```python
from build123d import *

# Parameters (mm, degrees)
F0_W     = 63.5
F0_H     = 63.5
F1_DEPTH = 3.175
F3_DEPTH = 25.4
F4_R     = 1.524
F6_D     = 8.4328


with BuildPart() as f1:
    # F0 (on Top) → F1 (new body)
    with BuildSketch(Plane.XY):
        with Locations((31.75, 31.75)):
            Rectangle(F0_W, F0_H)
    extrude(amount=F1_DEPTH)

    # F2 (on face) → F3 (join)
    with BuildSketch(Plane.XY.offset(3.175)):
        with BuildLine():
            ThreePointArc((31.75, 21.8313), (34.27345197, 22.87654803), (35.3187, 25.4))
            ThreePointArc((35.3187, 25.4), (29.22654803, 27.92345197), (31.75, 21.8313))
        make_face()
    extrude(amount=F3_DEPTH)

    # F4
    f4_edges = [f1.edges().sort_by_distance(p)[0] for p in [
        (31.75, 28.9687, 28.575),
    ]]
    fillet(f4_edges, radius=F4_R)

    # F6 (through all)
    with Locations(Plane.XY.offset(3.175)):
        with Locations((16.5602006018, 19.0660767257), (51.1259697378, 19.6664221585)):
            Hole(F6_D / 2)


solid = f1.part
```
Work out the finished part from the listing and answer in its coordinate system (mm). Round coordinates to 2 decimals unless told otherwise and drop trailing zeros. Loops run counter-clockwise (first coordinate to the right, second up) from the corner with the lowest first, then second, coordinate; pieces in that order, holes last. Notation, with made-up numbers: (68, 34.25) -> (123, 34.25) arc R21 ccw to (123, 53.25) -> close; hole circle Ø8 at (5.25, 34.25). An arc over 180 degrees is marked (long way). Write each question's results on one line, items separated by ' | '. Start each with the question number.
1. For a pull along X with two mould halves and no side action, classify faces 1 (the face through (31, 0, 2)), 2 (the face through (12.665, 17.451, 1.565)), 3 (the face through (63.5, 31, 2)) as +X half, -X half, draft (parallel to the pull), parting line (faces both ways), or undercut.
2. Section C-C (y = 32.5) is taken. Determine the outline of the cut face in (x, z) (3 decimals), plus the area to 3 significant figures.
3. Given pin 1 Ø3 at (y, z) = (9.5, 5.5) entering from -X; pin 2 Ø13.5 at (x, y) = (51.13, 19.67) entering from -Z; pin 3 Ø4 at (x, y) = (56, 19.5) entering from +Z (3 decimals); pin 4 Ø4 at (y, z) = (21.5, 9.5) entering from -X, each flat-ended and moving along its own axis, determine where each tip first touches the part or whether it passes through.
4. Find the intervals of material crossed by probe 1 along Z at (x, y) = (43, 31) (3 decimals); probe 2 along Y at (x, z) = (54, 1.75); probe 3 along X at (y, z) = (27, 4), in increasing order. Write a range as from..to.
5. Section A-A (x = 48) is taken. Determine the outline of the cut face in (y, z) (3 decimals), plus the area to 3 significant figures.
6. Section D-D (z = 12) is taken. Determine the outline of the cut face in (x, y).
7. Section B-B (y = 18) is taken. Determine the outline of the cut face in (x, z) (3 decimals).
Evaluation:
1) face 1: draft | face 2: undercut | face 3: +X half
2) outline: (0, 0) -> (63.5, 0) -> (63.5, 3.175) -> (0, 3.175) -> close | area: 202 mm2
3) pin 1: passes through | pin 2: stops at z = 0 | pin 3: stops at z = 3.175 | pin 4: stops at x = 28.73
4) probe 1: z = 0..3.175 | probe 2: y = 0..16.58, 22.75..63.5 | probe 3: x = 28.56..34.94
5) outline: (0, 0) -> (16.837, 0) -> (16.837, 3.175) -> (0, 3.175) -> close; (22.496, 0) -> (63.5, 0) -> (63.5, 3.175) -> (22.496, 3.175) -> close | area: 184 mm2
6) outline: circle Ø7.14 at (31.75, 25.4)
7) outline: (0, 0) -> (12.481, 0) -> (12.481, 3.175) -> (0, 3.175) -> close; (20.64, 0) -> (47.253, 0) -> (47.253, 3.175) -> (20.64, 3.175) -> close; (54.999, 0) -> (63.5, 0) -> (63.5, 3.175) -> (54.999, 3.175) -> close
